```python
from build123d import *

# Parameters (mm, degrees)
F0_R     = 12.7
F0_R_2   = 7.065837
F1_DEPTH = 50.8
F3_DEPTH = 80.772


with BuildPart() as f1:
    # F0 (on Front) → F1 (new body)
    with BuildSketch(Plane.XZ):
        Polygon((58.696682, 24.570704), (-54.328558, 24.570704), (-54.328558, 13.587744), (-54.328558, -13.587744), (-54.328558, -25.844741), (58.696682, -25.844741), align=None)
        with Locations((40.132153, -1.456042)):
            Circle(F0_R, mode=Mode.SUBTRACT)
        with Locations((-45.444705, 0)):
            Circle(F0_R_2, mode=Mode.SUBTRACT)
        with BuildLine():
            Line((-54.328558, -13.587744), (-54.328558, 13.587744))
            ThreePointArc((-54.328558, 13.587744), (-61.678917, 0), (-54.328558, -13.587744))
        make_face()
    extrude(amount=F1_DEPTH)

    # F2 (on face) → F3 (cut)
    with BuildSketch(Plane.YZ.offset(58.696682)):
        Polygon((-46.031717, 7.029241), (-35.797476, -10.768648), (-15.266932, -10.80448), (-4.970628, 6.957576), (-15.098626, 24.570704), (-35.863286, 24.570704), align=None)
    extrude(amount=-F3_DEPTH, mode=Mode.SUBTRACT)


solid = f1.part
```
Check sheet for the modelled part. Datum: model origin and axes. Units: mm. A direction names the side the tool comes from. Coordinates: 2 decimals unless noted, no trailing zeros. Write each loop counter-clockwise with the first axis right and the second up, starting at its lowest first coordinate (ties: lowest second). Pieces come first, ordered by that corner, then holes. Notation, with made-up numbers: M 87.25,-1 L 109.25,-1 A31 cw 109.25,25 Z; hole C -22.75,0.5 d3. An arc over 180 degrees is marked long. Write item = value, one per line. Start each with the question number.
1. Sectioned sample at A-A (y = -43.5). Record the cut outline in (x, z), then the cut area to 3 significant figures.
2. Thickness scan on probe 1 along X at (y, z) = (-41, -5); probe 2 along X at (y, z) = (-48, -15); probe 3 along Z at (x, y) = (19, -42.5). Record the ranges inside material, lowest first.
3. Tool access check on faces 4 (the flat face through (-54.329, -25, 19)), 5 (the cylindrical face through (37.379, -25.044, -13.854)), 6 (the flat face through (54.89, -10.19, -2.05)), 7 (the flat face through (-54.329, -25, -20)). Record the directions out of +Z, -Z, +X, -X, +Y, -Y that give a thin tool (end or side, any length) a straight path to the whole face; none if there is none.
4. Sectioned sample at B-B (x = 7.5). Record the cut outline in (y, z).
5. Sectioned sample at D-D (z = 21.5). Record the cut outline in (x, y), then the cut area to 3 significant figures.
6. Go/stop test with flat-tipped pins: pin 1 (6 mm diameter, centred on y = -16.5, z = 14, fed in from -X); pin 2 (3 mm diameter, centred on y = -29.5, z = 3.5, fed in from -X); pin 3 (3.5 mm diameter, centred on y = -35, z = 18.5, fed in from -X). Record where each tip stops, or that it passes through.
7. Sectioned sample at C-C (z = 0). Record the cut outline in (x, y), then the cut area to 3 significant figures.
8. Mould release check, pull along Y, two halves, no side actions. Record for faces 1 (the flat face through (18.88, -40.88, 15.92)), 2 (the flat face through (-2, -50.8, 0)), 3 (the flat face through (3, -36.3, 24.571)): pulls with the +Y half, pulls with the -Y half, needs draft (parallel to the pull), parting line crosses it, or undercut.
The answers:
q1.outline = M -54.33,-25.84 L 58.7,-25.84 L 58.7,2.63 L 52.16,2.63 A12.7 cw long 28.11,2.63 L -22.08,2.63 L -22.08,11.4 L 58.7,11.4 L 58.7,24.57 L -54.33,24.57 L -54.33,13.59 A16.23 ccw -54.33,-13.59 Z; hole C -45.44,0 d14.13
q1.area = 4,620 mm²
q2.probe_1 = -60.89 to -50.44, -40.45 to 27.94, 52.33 to 58.7
q2.probe_2 = -54.33 to 58.7
q2.probe_3 = -25.84 to 0.89, 13.12 to 24.57
q3.face_4 = +Z, -X, +Y, -Y
q3.face_5 = +Y, -Y
q3.face_6 = +X
q3.face_7 = -Z, -X, +Y, -Y
q4.outline = M -50.8,-25.84 L 0,-25.84 L 0,24.57 L -15.1,24.57 L -4.97,6.96 L -15.27,-10.8 L -35.8,-10.77 L -46.03,7.03 L -35.86,24.57 L -50.8,24.57 Z
q5.outline = M -54.33,-50.8 L 58.7,-50.8 L 58.7,-37.64 L -22.08,-37.64 L -22.08,-13.33 L 58.7,-13.33 L 58.7,0 L -54.33,0 Z
q5.area = 3,780 mm²
q6.pin_1 = -57.38
q6.pin_2 = -61.56
q6.pin_3 = -54.33
q7.outline = M -61.68,-50.8 L -52.51,-50.8 L -52.51,0 L -61.68,0 Z; M -38.38,-50.8 L 27.52,-50.8 L 27.52,-41.99 L -22.08,-41.99 L -22.08,-9 L 27.52,-9 L 27.52,0 L -38.38,0 Z; M 52.75,-50.8 L 58.7,-50.8 L 58.7,-41.99 L 52.75,-41.99 Z; M 52.75,-9 L 58.7,-9 L 58.7,0 L 52.75,0 Z
q7.area = 2,280 mm²
q8.face_1 = undercut
q8.face_2 = pulls with the -Y half
q8.face_3 = needs draft
